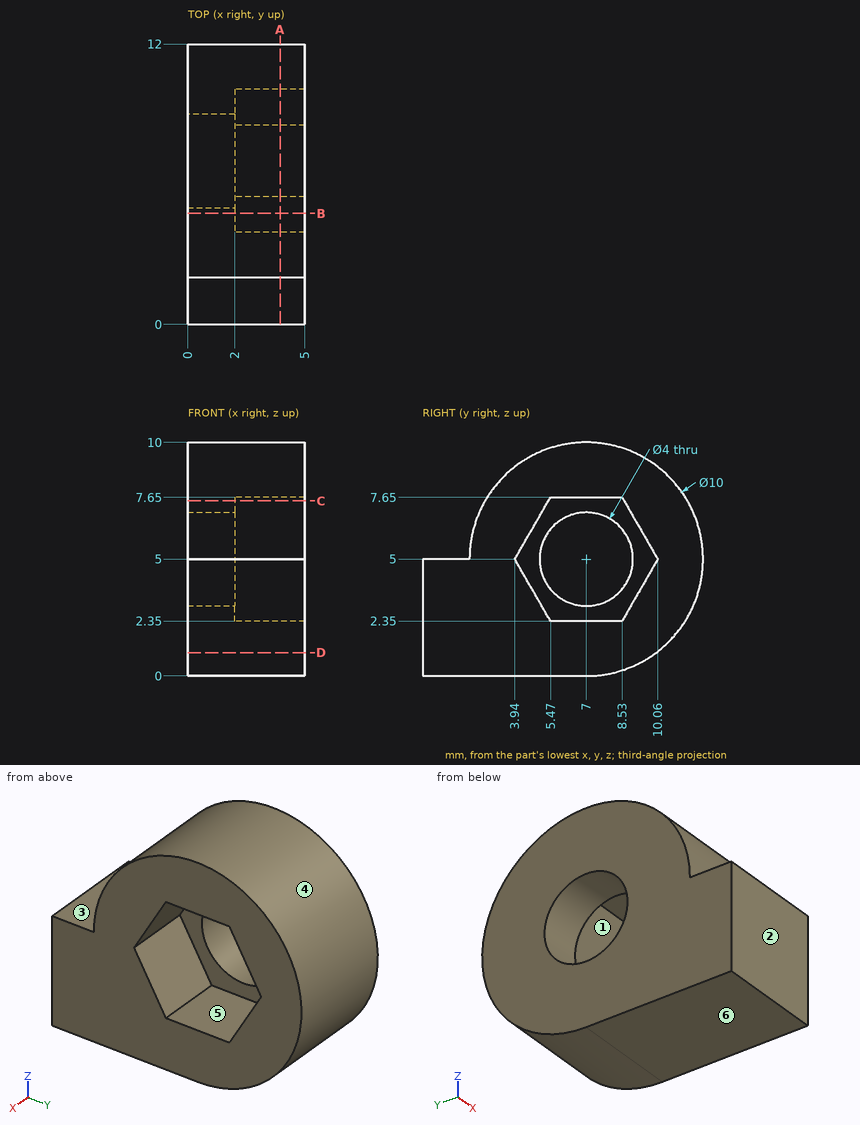
Study the drawing (mm; zero at the part's minimum x, y, z) and answer. A direction names the side the tool comes from. Give positions to 0.01 mm unless a question says otherwise; leave off trailing zeros. Order: outer loops, then holes, each group sorted by start corner. A loop starts at its lowest first (then second) coordinate and runs counter-clockwise, first axis right, second up.
1. Section B-B, the plane y = 4.75 is taken. Determine the outline of the cut face in (x, z).
Result sheet:
outline: (0, 0) - (5, 0) - (5, 3.6) - (2, 3.6) - (2, 6.4) - (5, 6.4) - (5, 9.47) - (0, 9.47) - close
2. The mould has two halves that part along Y. Classify the marked faces 4, 5 and 6: released by +Y, released by -Y, zero draft, split by the parting line, or undercut.
Result sheet:
face 4: split by the parting line
face 5: undercut
face 6: zero draft
3. Each of these flat-tipped pins is pushed along its axis until it touches: P1, Ø1, axis at x = 2, y = 1, coming from the +Z side; P2, Ø1.5, axis at x = 1, y = 2, coming from the +Z side. Where does it stop, or does it pass through?
Result sheet:
P1: stops at z = 5
P2: stops at z = 7.63
4. For the marked faces 1, 2 and 3, determine the directions among +Z, -Z, +X, -X, +Y, -Y from which every point of the face is accessible in a straight line to the end or side of a thin tool.
Result sheet:
face 1: +X
face 2: +Z, -Z, +X, -X, -Y
face 3: +Z, +X, -X, -Y
5. Straight lines are drawn through the part: L1, parallel to Z at x = 1.6, y = 7; L2, parallel to Y at x = 4.35, z = 3; L3, parallel to Z at x = 1.5, y = 6.25. For each, find the intervals that lie inside material, in ascending order.
Result sheet:
L1: z = 0 to 3, 7 to 10
L2: y = 0 to 5.09, 8.91 to 11.58
L3: z = 0 to 3.15, 6.85 to 9.94
6. Section D-D, the plane z = 1 is taken. Determine the outline of the cut face in (x, y), and give its area (3 significant figures).
Result sheet:
outline: (0, 0) - (5, 0) - (5, 10) - (0, 10) - close
area: 50.0 mm2
7. Section A-A, the plane x = 3.95 is taken. Determine the outline of the cut face in (y, z).
Result sheet:
outline: (0, 0) - (7, 0) arc R5 ccw (long way) to (2, 5) - (0, 5) - close; hole (3.94, 5) - (5.47, 2.35) - (8.53, 2.35) - (10.06, 5) - (8.53, 7.65) - (5.47, 7.65) - close
8. Section C-C, the plane z = 7.5 is taken. Determine the outline of the cut face in (x, y).
Result sheet:
outline: (0, 2.67) - (5, 2.67) - (5, 5.38) - (2, 5.38) - (2, 8.62) - (5, 8.62) - (5, 11.33) - (0, 11.33) - close
